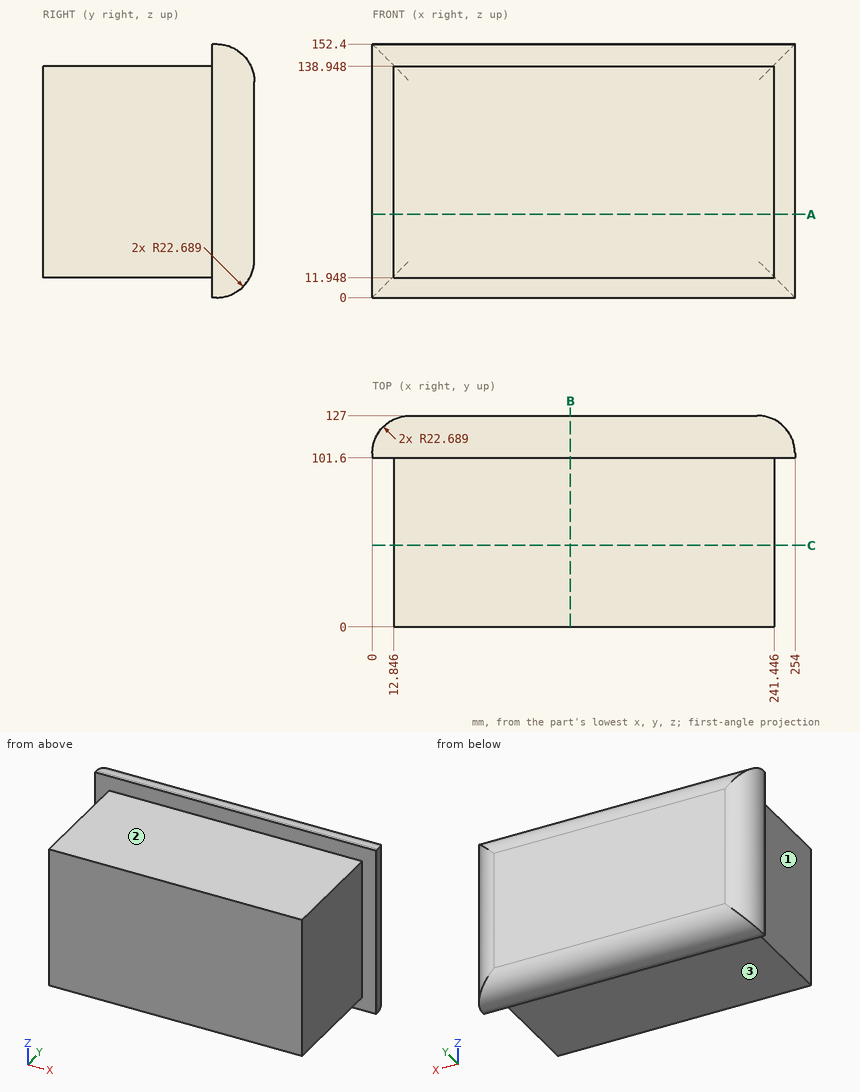
Here's the drawing with two shaded views (mm, measured from the low corner). I have some questions. A direction names the side the tool comes from. Round coordinates to 2 decimals unless told otherwise and drop trailing zeros. Order: outer loops, then holes, each group sorted by start corner. A loop starts at its lowest first (then second) coordinate and runs counter-clockwise, first axis right, second up. Notation, with made-up numbers: (86.5, 20.25) -> (114.5, 20.25) arc R18 cw to (114.5, 38.25) -> close; hole circle Ø3 at (-37.75, 18). An arc over 180 degrees is marked (long way). Return JSON: item names as keys, results as strings.
Q1. I need wall thicknesses on line 1 along X through (y, z) = (85, 13); line 2 along Z through (x, y) = (190, 14); line 3 along Y through (x, z) = (21, 61). Which ranges of each line are inside material? Lowest first, please. Write a range as from..to.
Filled sheet:
{"line 1": "x = 12.85..241.45", "line 2": "z = 11.95..138.95", "line 3": "y = 0..126.94"}
Q2. If we section it at A-A on z = 50: List the corners of the cut face in (x, y) for me.
Filled sheet:
{"outline": "(0, 101.6) -> (12.85, 101.6) -> (12.85, 0) -> (241.45, 0) -> (241.45, 101.6) -> (254, 101.6) -> (254, 104.31) arc R22.69 ccw to (231.31, 127) -> (22.69, 127) arc R22.69 ccw to (0, 104.31) -> close"}
Q3. If we section it at C-C on y = 49: List the corners of the cut face in (x, z) for me, plus the area to 3 significant figures.
Filled sheet:
{"outline": "(12.85, 11.95) -> (241.45, 11.95) -> (241.45, 138.95) -> (12.85, 138.95) -> close", "area": "29,000 mm^2"}
Q4. If we section it at B-B on x = 119: List the corners of the cut face in (y, z) for me, plus the area to 3 significant figures.
Filled sheet:
{"outline": "(0, 11.95) -> (101.6, 11.95) -> (101.6, 0) -> (104.31, 0) arc R22.69 ccw to (127, 22.69) -> (127, 129.71) arc R22.69 ccw to (104.31, 152.4) -> (101.6, 152.4) -> (101.6, 138.95) -> (0, 138.95) -> close", "area": "16,600 mm^2"}
Q5. Which directions (+Z, -Z, +X, -X, +Y, -Y) give clear straight access to the entire face, cutting with the end or side of a thin tool? Please do the marked faces 1, 2 and 3.
Filled sheet:
{"face 1": "+Z, -Z, -X, -Y", "face 2": "+Z, +X, -X, -Y", "face 3": "-Z, +X, -X, -Y"}
Q6. For pin 1 Ø3 at (y, z) = (74.5, 78) entering from +X; pin 2 Ø8 at (x, y) = (33.5, 70.5) entering from -Z; pin 3 Ø2 at (x, z) = (197, 131.5) entering from +Y, each with a flat end and sliding along its axis, tell me the tip position at first contact or that it passes through.
Filled sheet:
{"pin 1": "stops at x = 241.45", "pin 2": "stops at z = 11.95", "pin 3": "stops at y = 126.99"}
